from build123d import *

# Parameters (mm, degrees)
ESQUISSE1_R             = 40
BOSS_EXTRU_1_DEPTH      = 24
ESQUISSE6_R             = 33.5
ENL_V_MAT_EXTRU_5_DEPTH = 8
ENL_V_START             = -8
ESQUISSE3_R             = 33.5
ENL_V_MAT_EXTRU_6_DEPTH = 8
CONG_12_R               = 12
CONG_16_R               = 12
ESQUISSE11_R            = 33.5
ESQUISSE11_R_2          = 26.5
BOSS_EXTRU_3_DEPTH      = 8
BOSS_EXTRU_4_START      = 8
ESQUISSE13_R            = 33.5
ESQUISSE13_R_2          = 26.5
BOSS_EXTRU_4_DEPTH      = 8
ESQUISSE14_R            = 3.5
ESQUISSE14_R_2          = 2
ENL_V_MAT_EXTRU_7_DEPTH = 59.787753827


with BuildPart() as part:
    # Esquisse1 → Boss.-Extru.1 (new body)
    with BuildSketch(Plane.XY):
        Circle(ESQUISSE1_R)
    extrude(amount=BOSS_EXTRU_1_DEPTH)

    # Esquisse6 → Enlèv. mat.-Extru.5 (cut)
    with BuildSketch(Plane(origin=(0, 0, 0), x_dir=(-1, 0, 0), z_dir=(0, 0, -1))):
        Circle(ESQUISSE6_R)
    extrude(amount=-ENL_V_MAT_EXTRU_5_DEPTH, mode=Mode.SUBTRACT)

    # Esquisse3 → Enlèv. mat.-Extru.6 (cut)
    with BuildSketch(Plane.XY.offset(24).offset(ENL_V_START)):
        with Locations(Location((0, 0, 0), (0, 0, 180))):
            Circle(ESQUISSE3_R)
    extrude(amount=ENL_V_MAT_EXTRU_6_DEPTH, mode=Mode.SUBTRACT)

    # Congé12
    # the kernel refuses this fillet: 12 mm, written as the material it takes off along each edge
    with BuildSketch(Plane(origin=(0, 0, 0), x_dir=(1, 0, 0), z_dir=(0, -1, 0))) as cong_12_piece_1:
        with BuildLine():
            CenterArc((28, 10.665364504), CONG_12_R, 297.279612736, 62.720387264)
            Line((33.5, 0), (33.61, -0.21330729))
            ThreePointArc((33.61, -0.21330729), (36.75, -0.24), (40, -0.24))
            Line((40, -0.24), (40.24, 0))
            Line((40.24, 0), (40.24, 10.665364504))
            Line((40.24, 10.665364504), (40, 10.665364504))
        make_face()
    revolve(axis=Axis((0, 0, 0), (0, 0, 1)), mode=Mode.SUBTRACT)

    # Congé16
    # the kernel refuses this fillet: 12 mm, written as the material it takes off along each edge
    with BuildSketch(Plane(origin=(0, 0, 24), x_dir=(1, 0, 0), z_dir=(0, -1, 0))) as cong_16_piece_1:
        with BuildLine():
            CenterArc((28, -10.665364504), CONG_16_R, 0, 62.720387264)
            Line((33.5, 0), (33.61, 0.21330729))
            ThreePointArc((33.61, 0.21330729), (36.75, 0.24), (40, 0.24))
            Line((40, 0.24), (40.24, 0))
            Line((40.24, 0), (40.24, -10.665364504))
            Line((40.24, -10.665364504), (40, -10.665364504))
        make_face()
    revolve(axis=Axis((0, 0, 24), (0, 0, 1)), mode=Mode.SUBTRACT)

    # Esquisse11 → Boss.-Extru.3 (add)
    with BuildSketch(Plane.XY.offset(16)):
        with Locations(Location((0, 0, 0), (0, 0, 180))):
            Circle(ESQUISSE11_R)
        Circle(ESQUISSE11_R_2, mode=Mode.SUBTRACT)
    extrude(amount=BOSS_EXTRU_3_DEPTH)

    # Esquisse13 → Boss.-Extru.4 (add)
    with BuildSketch(Plane(origin=(0, 0, 8), x_dir=(-1, 0, 0), z_dir=(0, 0, -1)).offset(BOSS_EXTRU_4_START)):
        Circle(ESQUISSE13_R)
        with Locations(Location((0, 0, 0), (0, 0, 180))):
            Circle(ESQUISSE13_R_2, mode=Mode.SUBTRACT)
    extrude(amount=-BOSS_EXTRU_4_DEPTH)

    # Esquisse14 → Enlèv. mat.-Extru.7 (cut, through all)
    with BuildSketch(Plane(origin=(0, 0, 8), x_dir=(-1, 0, 0), z_dir=(0, 0, -1))):
        Circle(ESQUISSE14_R)
        with Locations((-8.5, 0)):
            Circle(ESQUISSE14_R_2)
        with Locations((-19, 0)):
            Circle(ESQUISSE14_R)
        with Locations((0, 8.5)):
            Circle(ESQUISSE14_R_2)
        with Locations((8.5, 0)):
            Circle(ESQUISSE14_R_2)
        with Locations((0, -8.5)):
            Circle(ESQUISSE14_R_2)
        with Locations((-13.435028843, 13.435028843)):
            Circle(ESQUISSE14_R)
        with Locations((0, 19)):
            Circle(ESQUISSE14_R)
        with Locations((13.435028843, 13.435028843)):
            Circle(ESQUISSE14_R)
        with Locations((19, 0)):
            Circle(ESQUISSE14_R)
        with Locations((13.435028843, -13.435028843)):
            Circle(ESQUISSE14_R)
        with Locations((0, -19)):
            Circle(ESQUISSE14_R)
        with Locations((-13.435028843, -13.435028843)):
            Circle(ESQUISSE14_R)
    extrude(amount=-ENL_V_MAT_EXTRU_7_DEPTH, mode=Mode.SUBTRACT)


solid = part.part
For this review, take the finished solid that the model builds, in its own axes (mm). A direction names the side the tool comes from. Give positions to 0.01 mm unless a question says otherwise; leave off trailing zeros. Loops run counter-clockwise (first coordinate to the right, second up) from the corner with the lowest first, then second, coordinate; pieces in that order, holes last.
Item 1: Insertion check: pin 1 (6 mm diameter, centred on y = 26.5, z = 19, fed in from +X); pin 2 (3 mm diameter, centred on y = -6.5, z = 8, fed in from +X); pin 3 (2.5 mm diameter, centred on x = 0, y = -8.5, fed in from +Z); pin 4 (11 mm diameter, centred on x = -13.44, y = 13.44, fed in from +Z). Each pin has a flat end and moves straight along its axis. Give the tip position at first contact, or say it passes through.
Item 2: Take a section at D-D, the plane z = 2.75. State the section outline as (x, y) points.
Item 3: Tool access review of faces 1 (the flat face through (0, -6, 8)), 2 (the cylindrical face through (10.1, -1.2, 11.9)), 3 (the flat face through (0, 6, 16)): name each direction out of +Z, -Z, +X, -X, +Y, -Y from which nothing blocks a thin tool from reaching the whole face with its end or side.
Item 4: Take a section at A-A, the plane z = 11.75. Give the number of separate pieces and of enclosed holes in the cut face, and give its area (3 significant figures).
Item 5: For line 1 along Y through (x, z) = (0, 13.75); line 2 along Z through (x, y) = (-16.5, 6); line 3 along X through (y, z) = (22, 18.25), list the stretches that pass through material, from the lowest coordinate up.
Item 6: Draft analysis for pull direction X (two halves, no side actions). For faces 4 (the flat face through (-25, 10, 0)), 5 (the cylindrical face through (-8.67, -39.05, 11.98)), 6 (the cylindrical face through (-22.34, 1.05, 11.94)), state which applies: +X half, -X half, draft (parallel to the pull), parting line (faces both ways), or undercut.
Calculated:
1. pin 1: stops at x = 31.14
1. pin 2: stops at x = 39.52
1. pin 3: passes through
1. pin 4: stops at z = 16
2. outline: circle Ø74.04 at (0, 0); hole circle Ø53 at (0, 0)
3. face 1: -Z
3. face 2: +Z, -Z
3. face 3: +Z
4. separate pieces: 1
4. enclosed holes: 13
4. area: 4,630 mm2
5. line 1: y = -39.99 to -22.5, -15.5 to -10.5, -6.5 to -3.5, 3.5 to 6.5, 10.5 to 15.5, 22.5 to 39.99
5. line 2: z = 8 to 16
5. line 3: x = -32.14 to -14.77, 14.77 to 32.14
6. face 4: draft
6. face 5: parting line
6. face 6: undercut
